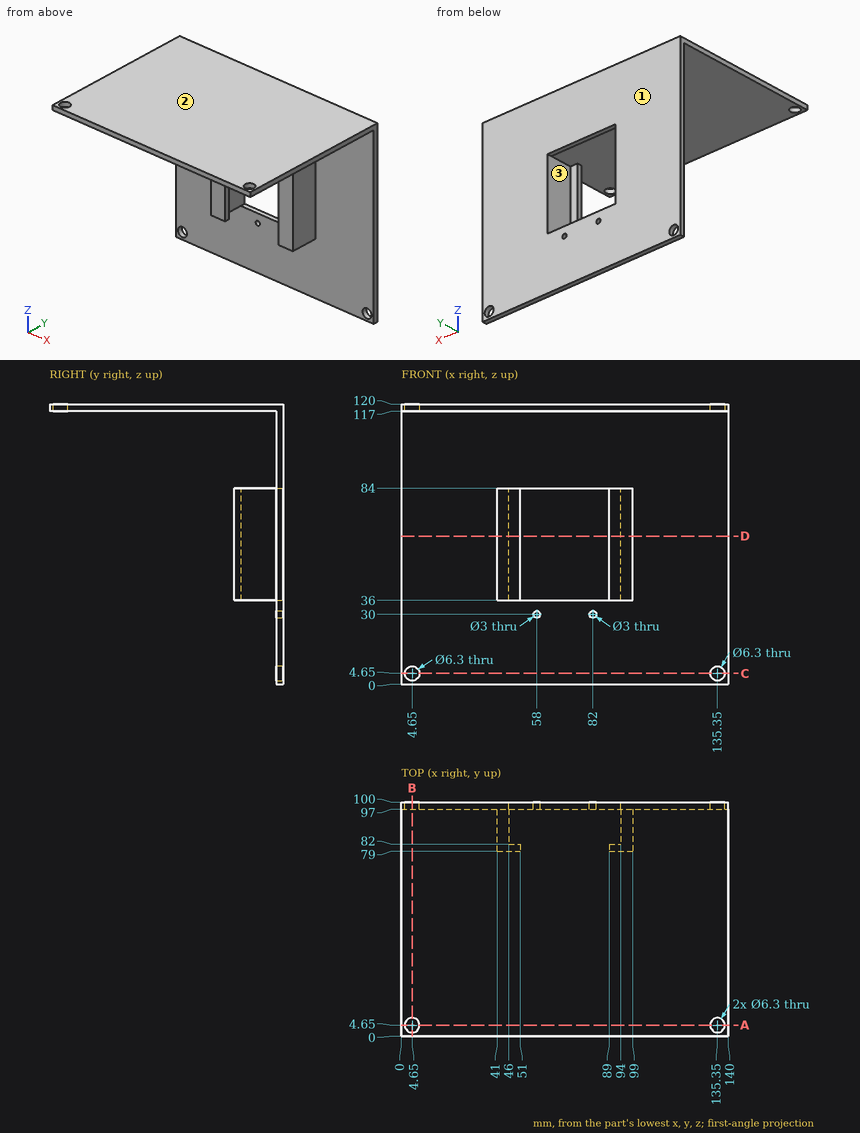
Verification items for this drawing (mm, ordinates from the low corner). Give positions to 0.01 mm unless a question says otherwise; leave off trailing zeros. Loops run counter-clockwise (first coordinate to the right, second up) from the corner with the lowest first, then second, coordinate; pieces in that order, holes last.
1. Cross-section at A-A on y = 4.65. Record the cut outline in (x, z).
Derived:
outline: (0, 117) - (1.5, 117) - (1.5, 120) - (0, 120) - close; (7.8, 117) - (132.2, 117) - (132.2, 120) - (7.8, 120) - close; (138.5, 117) - (140, 117) - (140, 120) - (138.5, 120) - close
2. Material ranges on probe 1 along X at (y, z) = (98, 30); probe 2 along X at (y, z) = (99.25, 4.65); probe 3 along Y at (x, z) = (135.35, 118), recorded low to high.
Derived:
probe 1: x = 0 to 56.5, 59.5 to 80.5, 83.5 to 140
probe 2: x = 0 to 1.5, 7.8 to 132.2, 138.5 to 140
probe 3: y = 0 to 1.5, 7.8 to 100
3. Go/stop test with flat-tipped pins: P1, Ø1, axis at x = 125, z = 36.5, coming from the -Y side; P2, Ø5, axis at x = 93, z = 51, coming from the -Y side; P3, Ø9, axis at y = 87.5, z = 67.5, coming from the +X side. Record where each tip stops, or that it passes through.
Derived:
P1: stops at y = 97
P2: stops at y = 79
P3: stops at x = 99
4. Release check for a two-part mould opening along Z. For the marked faces 1, 2 and 3 record: +Z half, -Z half, draft (parallel to the pull), parting line (faces both ways), or undercut.
Derived:
face 1: draft
face 2: +Z half
face 3: undercut
5. Cross-section at B-B on x = 4.65. Record the cut outline in (y, z).
Derived:
outline: (0, 117) - (1.5, 117) - (1.5, 120) - (0, 120) - close; (7.8, 117) - (97, 117) - (97, 7.8) - (100, 7.8) - (100, 120) - (7.8, 120) - close; (97, 0) - (100, 0) - (100, 1.5) - (97, 1.5) - close
6. Cross-section at C-C on z = 4.65. Record the cut outline in (x, y).
Derived:
outline: (0, 97) - (1.5, 97) - (1.5, 100) - (0, 100) - close; (7.8, 97) - (132.2, 97) - (132.2, 100) - (7.8, 100) - close; (138.5, 97) - (140, 97) - (140, 100) - (138.5, 100) - close
7. Cross-section at D-D on z = 63.5. Record the cut outline in (x, y), and give its area (3 significant figures).
Derived:
outline: (0, 97) - (41, 97) - (41, 79) - (51, 79) - (51, 82) - (46, 82) - (46, 100) - (0, 100) - close; (89, 79) - (99, 79) - (99, 97) - (140, 97) - (140, 100) - (94, 100) - (94, 82) - (89, 82) - close
area: 486 mm2
